```python
from build123d import *

# Parameters (mm, degrees)
SKETCH001_W  = 85
SKETCH001_H  = 74
SKETCH001_R  = 1.5
PAD_DEPTH    = 1.5
FILLET_R     = 2
SKETCH_W     = 27
SKETCH_H     = 1.5
PAD001_DEPTH = 2


with BuildPart() as part:
    # Sketch001 → Pad (new body)
    with BuildSketch(Plane.XY):
        Rectangle(SKETCH001_W, SKETCH001_H)
        with Locations((-27, 24)):
            Circle(SKETCH001_R, mode=Mode.SUBTRACT)
        with Locations((-9, 24)):
            Circle(SKETCH001_R, mode=Mode.SUBTRACT)
        with Locations((9, 24)):
            Circle(SKETCH001_R, mode=Mode.SUBTRACT)
        with Locations((27, 24)):
            Circle(SKETCH001_R, mode=Mode.SUBTRACT)
        with Locations((-27, 12)):
            Circle(SKETCH001_R, mode=Mode.SUBTRACT)
        with Locations((-9, 12)):
            Circle(SKETCH001_R, mode=Mode.SUBTRACT)
        with Locations((9, 12)):
            Circle(SKETCH001_R, mode=Mode.SUBTRACT)
        with Locations((27, 12)):
            Circle(SKETCH001_R, mode=Mode.SUBTRACT)
        with Locations((-27, 0)):
            Circle(SKETCH001_R, mode=Mode.SUBTRACT)
        with Locations((-9, 0)):
            Circle(SKETCH001_R, mode=Mode.SUBTRACT)
        with Locations((9, 0)):
            Circle(SKETCH001_R, mode=Mode.SUBTRACT)
        with Locations((27, 0)):
            Circle(SKETCH001_R, mode=Mode.SUBTRACT)
        with Locations((-27, -12)):
            Circle(SKETCH001_R, mode=Mode.SUBTRACT)
        with Locations((-9, -12)):
            Circle(SKETCH001_R, mode=Mode.SUBTRACT)
        with Locations((9, -12)):
            Circle(SKETCH001_R, mode=Mode.SUBTRACT)
        with Locations((27, -12)):
            Circle(SKETCH001_R, mode=Mode.SUBTRACT)
        with Locations((-27, -24)):
            Circle(SKETCH001_R, mode=Mode.SUBTRACT)
        with Locations((-9, -24)):
            Circle(SKETCH001_R, mode=Mode.SUBTRACT)
        with Locations((9, -24)):
            Circle(SKETCH001_R, mode=Mode.SUBTRACT)
        with Locations((27, -24)):
            Circle(SKETCH001_R, mode=Mode.SUBTRACT)
    extrude(amount=PAD_DEPTH)

    # Fillet
    fillet_edges = [part.edges().sort_by_distance(p)[0] for p in [
        (-42.5, 37, 0.75),
        (42.5, -37, 0.75),
        (-42.5, -37, 0.75),
        (42.5, 37, 0.75),
    ]]
    fillet(fillet_edges, radius=FILLET_R)

    # Sketch (on Face2 of Fillet) → Pad001 (join)
    with BuildSketch(Plane(origin=(0, 0, 0), x_dir=(1, 0, 0), z_dir=(0, 0, -1))):
        with Locations((-26, -34)):
            Rectangle(SKETCH_W, SKETCH_H)
    extrude(amount=PAD001_DEPTH)


solid = part.part
```
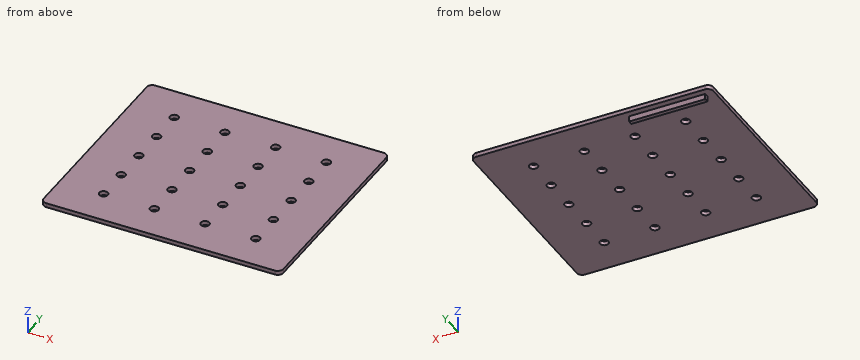
Can you work these out from the model? Positions are in its coordinate system, mm. Coordinates: 2 decimals unless noted, no trailing zeros. Order: outer loops, then holes, each group sorted by start corner. A loop starts at its lowest first (then second) coordinate and runs counter-clockwise, first axis right, second up.
1. If we section it at C-C (x = -14.5): Please give me the cut outline in (y, z), then the cut area to 3 significant figures.
2. I'm going to push flat-ended pins straight in: pin 1 (5 mm diameter, centred on x = -9, y = 12, fed in from +Z); pin 2 (4 mm diameter, centred on x = -9, y = -12, fed in from -Z). Where does each tip first touch, or does it pass through?
3. If we section it at D-D (z = -0.9): Please give me the cut outline in (x, y), then the cut area to 3 significant figures.
4. If we section it at B-B (y = 12): Please give me the cut outline in (x, z).
5. If we section it at A-A (x = -27): Please give me the cut outline in (y, z), then the cut area to 3 significant figures.
6. I need wall thicknesses on line 1 (Y direction, x = -27, z = 0.9); line 2 (Z direction, x = -4, y = 8); line 3 (Y direction, x = -31, z = -1.45). Which ranges of each line are inside material? Lowest first, please.
Entries:
1. outline: (-37, 0) - (33.25, 0) - (33.25, -2) - (34.75, -2) - (34.75, 0) - (37, 0) - (37, 1.5) - (-37, 1.5) - close
1. area: 114 mm2
2. pin 1: stops at z = 1.5
2. pin 2: stops at z = 0
3. outline: (-39.5, 33.25) - (-12.5, 33.25) - (-12.5, 34.75) - (-39.5, 34.75) - close
3. area: 40.5 mm2
4. outline: (-42.5, 0) - (-28.5, 0) - (-28.5, 1.5) - (-42.5, 1.5) - close; (-25.5, 0) - (-10.5, 0) - (-10.5, 1.5) - (-25.5, 1.5) - close; (-7.5, 0) - (7.5, 0) - (7.5, 1.5) - (-7.5, 1.5) - close; (10.5, 0) - (25.5, 0) - (25.5, 1.5) - (10.5, 1.5) - close; (28.5, 0) - (42.5, 0) - (42.5, 1.5) - (28.5, 1.5) - close
5. outline: (-37, 0) - (-25.5, 0) - (-25.5, 1.5) - (-37, 1.5) - close; (-22.5, 0) - (-13.5, 0) - (-13.5, 1.5) - (-22.5, 1.5) - close; (-10.5, 0) - (-1.5, 0) - (-1.5, 1.5) - (-10.5, 1.5) - close; (1.5, 0) - (10.5, 0) - (10.5, 1.5) - (1.5, 1.5) - close; (13.5, 0) - (22.5, 0) - (22.5, 1.5) - (13.5, 1.5) - close; (25.5, 0) - (33.25, 0) - (33.25, -2) - (34.75, -2) - (34.75, 0) - (37, 0) - (37, 1.5) - (25.5, 1.5) - close
5. area: 91.5 mm2
6. line 1: y = -37 to -25.5, -22.5 to -13.5, -10.5 to -1.5, 1.5 to 10.5, 13.5 to 22.5, 25.5 to 37
6. line 2: z = 0 to 1.5
6. line 3: y = 33.25 to 34.75
